Check sheet for the drawn part. Datum: minimum x, y, z corner. Units: mm. A direction names the side the tool comes from. Round coordinates to 2 decimals unless told otherwise and drop trailing zeros. Write each loop counter-clockwise with the first axis right and the second up, starting at its lowest first coordinate (ties: lowest second). Pieces come first, ordered by that corner, then holes. Notation, with made-up numbers: (-29.75, 23.5) - (-16.75, 23.5) arc R15 ccw to (-16.75, 44.5) - close; hole circle Ø5 at (58.5, 61). An arc over 180 degrees is marked (long way). Answer as a JSON object with one key per item and string values.
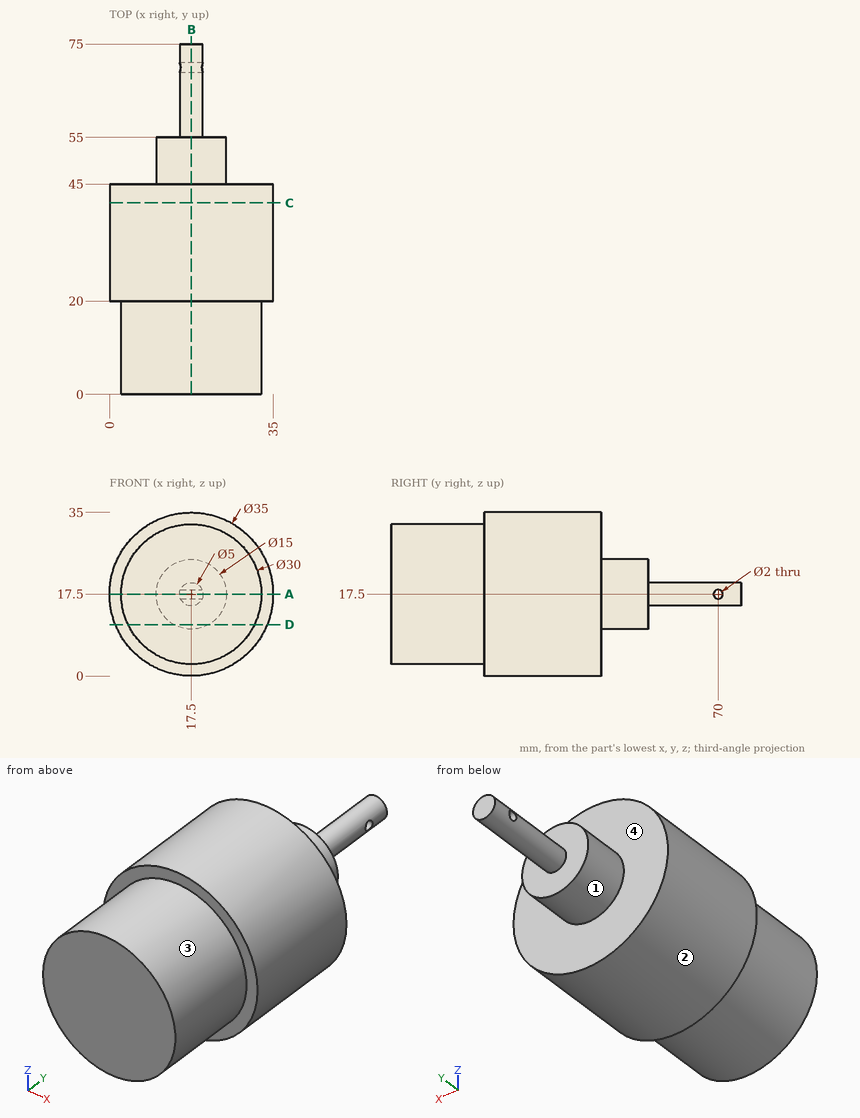
1. Access from +Z, -Z, +X, -X, +Y, -Y to the whole of each face (thin tool, end or side, straight path). Record for the marked faces 1 and 2.
Completed:
{"face 1": "+Y", "face 2": "+Y, -Y"}
2. Material ranges on probe 1 along Z at (x, y) = (17.5, 70); probe 2 along Y at (x, z) = (16.2, 17.5); probe 3 along Y at (x, z) = (19.5, 15), recorded low to high. Write a range as from..to.
Completed:
{"probe 1": "z = 15..16.5, 18.5..20", "probe 2": "y = 0..69, 71..75", "probe 3": "y = 0..55"}
3. Cross-section at A-A (z = 17.5). Record the boundary of the cut face in (x, y).
Completed:
{"outline": "(0, 20) - (2.5, 20) - (2.5, 0) - (32.5, 0) - (32.5, 20) - (35, 20) - (35, 45) - (25, 45) - (25, 55) - (20, 55) - (20, 69) - (15, 69) - (15, 55) - (10, 55) - (10, 45) - (0, 45) - close; (15, 71) - (20, 71) - (20, 75) - (15, 75) - close"}
4. Go/stop test with flat-tipped pins: pin 1 (4 mm diameter, centred on x = 16.5, z = 12, fed in from +Y); pin 2 (5 mm diameter, centred on x = 21, y = 9, fed in from +Z); pin 3 (2 mm diameter, centred on x = 25, y = 26, fed in from -Z). Record where each tip stops, or that it passes through.
Completed:
{"pin 1": "stops at y = 55", "pin 2": "stops at z = 32.47", "pin 3": "stops at z = 1.25"}
5. Cross-section at D-D (z = 11). Record the boundary of the cut face in (x, y).
Completed:
{"outline": "(1.25, 20) - (3.98, 20) - (3.98, 0) - (31.02, 0) - (31.02, 20) - (33.75, 20) - (33.75, 45) - (21.24, 45) - (21.24, 55) - (13.76, 55) - (13.76, 45) - (1.25, 45) - close"}
6. Cross-section at B-B (x = 17.5). Record the boundary of the cut face in (y, z).
Completed:
{"outline": "(0, 2.5) - (20, 2.5) - (20, 0) - (45, 0) - (45, 10) - (55, 10) - (55, 15) - (75, 15) - (75, 20) - (55, 20) - (55, 25) - (45, 25) - (45, 35) - (20, 35) - (20, 32.5) - (0, 32.5) - close; hole circle Ø2 at (70, 17.5)"}
7. Mould release check, pull along X, two halves, no side actions. Record for the marked faces 3 and 4: released by +X, released by -X, zero draft, split by the parting line, or undercut.
Completed:
{"face 3": "split by the parting line", "face 4": "zero draft"}
8. Cross-section at C-C (y = 41). Record the boundary of the cut face in (x, z).
Completed:
{"outline": "circle Ø35 at (17.5, 17.5)"}
